```python
from build123d import *

# Parameters (mm, degrees)
SKETCH1_R           = 32.5
BOSS_EXTRUDE1_DEPTH = 2
CUT_EXTRUDE2_DEPTH  = 47.005434462
SKETCH2_R           = 2.5
CUT_EXTRUDE1_DEPTH  = 47.005434462
SKETCH5_R           = 1.5
CUT_EXTRUDE3_DEPTH  = 10


with BuildPart() as part:
    # Sketch1 → Boss-Extrude1 (new body)
    with BuildSketch(Plane(origin=(0, 0, 0), x_dir=(1, 0, 0), z_dir=(0, 1, 0))):
        with Locations(Location((0, 0, 0), (0, 0, 270))):
            Circle(SKETCH1_R)
    extrude(amount=BOSS_EXTRUDE1_DEPTH)

    # Sketch4 → Cut-Extrude2 (cut, through all)
    with BuildSketch(Plane(origin=(0, 2, 0), x_dir=(1, 0, 0), z_dir=(0, 1, 0))):
        with BuildLine():
            Line((-3, -2.645751311), (-3, 2.645751311))
            ThreePointArc((-3, 2.645751311), (4, 0), (-3, -2.645751311))
        make_face()
    extrude(amount=-CUT_EXTRUDE2_DEPTH, mode=Mode.SUBTRACT)

    # Sketch2 → Cut-Extrude1 (cut, through all)
    with BuildSketch(Plane(origin=(0, 2, 0), x_dir=(1, 0, 0), z_dir=(0, 1, 0))):
        with Locations((-30.026084807, -12.437211552)):
            Circle(SKETCH2_R)
        with Locations((-32.5, 0)):
            Circle(SKETCH2_R)
        with Locations((-31.875521613, 6.340435466)):
            Circle(SKETCH2_R)
        with Locations((-30.026084807, 12.437211552)):
            Circle(SKETCH2_R)
        with Locations((-27.0227624, 18.056032573)):
            Circle(SKETCH2_R)
        with Locations((-22.980970389, 22.980970389)):
            Circle(SKETCH2_R)
        with Locations((-18.056032573, 27.0227624)):
            Circle(SKETCH2_R)
        with Locations((-12.437211552, 30.026084807)):
            Circle(SKETCH2_R)
        with Locations((-6.340435466, 31.875521613)):
            Circle(SKETCH2_R)
        with Locations((0, 32.5)):
            Circle(SKETCH2_R)
        with Locations((6.340435466, 31.875521613)):
            Circle(SKETCH2_R)
        with Locations((12.437211552, 30.026084807)):
            Circle(SKETCH2_R)
        with Locations((18.056032573, 27.0227624)):
            Circle(SKETCH2_R)
        with Locations((22.980970389, 22.980970389)):
            Circle(SKETCH2_R)
        with Locations((27.0227624, 18.056032573)):
            Circle(SKETCH2_R)
        with Locations((30.026084807, 12.437211552)):
            Circle(SKETCH2_R)
        with Locations((31.875521613, 6.340435466)):
            Circle(SKETCH2_R)
        with Locations((32.5, 0)):
            Circle(SKETCH2_R)
        with Locations((31.875521613, -6.340435466)):
            Circle(SKETCH2_R)
        with Locations((30.026084807, -12.437211552)):
            Circle(SKETCH2_R)
        with Locations((27.0227624, -18.056032573)):
            Circle(SKETCH2_R)
        with Locations((22.980970389, -22.980970389)):
            Circle(SKETCH2_R)
        with Locations((18.056032573, -27.0227624)):
            Circle(SKETCH2_R)
        with Locations((12.437211552, -30.026084807)):
            Circle(SKETCH2_R)
        with Locations((6.340435466, -31.875521613)):
            Circle(SKETCH2_R)
        with Locations((0, -32.5)):
            Circle(SKETCH2_R)
        with Locations((-6.340435466, -31.875521613)):
            Circle(SKETCH2_R)
        with Locations((-12.437211552, -30.026084807)):
            Circle(SKETCH2_R)
        with Locations((-18.056032573, -27.0227624)):
            Circle(SKETCH2_R)
        with Locations((-22.980970389, -22.980970389)):
            Circle(SKETCH2_R)
        with Locations((-27.0227624, -18.056032573)):
            Circle(SKETCH2_R)
        with Locations((-31.875521613, -6.340435466)):
            Circle(SKETCH2_R)
    extrude(amount=-CUT_EXTRUDE1_DEPTH, mode=Mode.SUBTRACT)

    # Sketch5 → Cut-Extrude3 (cut)
    with BuildSketch(Plane(origin=(0, 2, 0), x_dir=(1, 0, 0), z_dir=(0, 1, 0))):
        with Locations(Location((-25, 0, 0), (0, 0, 270))):
            Circle(SKETCH5_R)
        with Locations(Location((12.5, 21.650635095, 0), (0, 0, 270))):
            Circle(SKETCH5_R)
        with Locations(Location((12.5, -21.650635095, 0), (0, 0, 270))):
            Circle(SKETCH5_R)
    extrude(amount=-CUT_EXTRUDE3_DEPTH, mode=Mode.SUBTRACT)


solid = part.part
```
Here's how the part is built. I have some questions about the finished solid (model axes, mm). Give positions to 0.01 mm unless a question says otherwise; leave off trailing zeros. Order: outer loops, then holes, each group sorted by start corner. A loop starts at its lowest first (then second) coordinate and runs counter-clockwise, first axis right, second up. Notation, with made-up numbers: (-5.5, 22.5) -> (20.5, 22.5) arc R9 ccw to (20.5, 34.5) -> close; hole circle Ø1 at (17, 68.25). An arc over 180 degrees is marked (long way). Use CSV: the item, a comma, the result in double quotes. Start each with the question number.
Item 1: Suppose I cut it at D-D (x = -13.5). List the corners of the cut face in (y, z) for me, and give its area (3 significant figures).
Item 2: Thinking about a two-plate mould opening in Z: for faces 1 (the flat face through (0, 2, 7)), 2 (the cylindrical face through (29.435, 1.014, 5.8)), 3 (the cylindrical face through (0, 1, 30)), which applies, pulls with the +Z half, pulls with the -Z half, needs draft (parallel to the pull), parting line crosses it, or undercut?
Item 3: I'm going to push flat-ended pins straight in: P1, Ø1.8, axis at x = 12.5, z = -21.65, coming from the +Y side; P2, Ø6, axis at x = -12.5, z = -13, coming from the -Y side; P3, Ø0.6, axis at y = 1, z = 0, coming from the +X side. Where does each tip first touch, or does it pass through?
Item 4: Suppose I cut it at C-C (y = 0.55). Give the number of separate pieces and of enclosed holes in the cut face, and give its area (3 significant figures).
Item 5: Suppose I cut it at A-A (z = 0). List the corners of the cut face in (x, y) for me, and give its area (3 significant figures).
Item 6: If I drill on probe 1 along X at (y, z) = (0.9, 0); probe 2 along X at (y, z) = (1.65, 21); probe 3 along Z at (x, y) = (0, 0.85), over which ranges is the centre line in solid material (lowest first)? Write a range as [from, to].
Item 7: Suppose I cut it at B-B (x = 12.5). List the corners of the cut face in (y, z) for me.
Answer block:
1,outline,"(0, -27.76) -> (2, -27.76) -> (2, 27.76) -> (0, 27.76) -> close"
1,area,"111 mm^2"
2,face 1,"needs draft"
2,face 2,"undercut"
2,face 3,"pulls with the +Z half"
3,P1,"passes through"
3,P2,"stops at y = 0"
3,P3,"stops at x = 30.02"
4,separate pieces,"1"
4,enclosed holes,"4"
4,area,"2,940 mm^2"
5,outline,"(-30, 0) -> (-26.5, 0) -> (-26.5, 2) -> (-30, 2) -> close; (-23.5, 0) -> (-3, 0) -> (-3, 2) -> (-23.5, 2) -> close; (4, 0) -> (30, 0) -> (30, 2) -> (4, 2) -> close"
5,area,"100 mm^2"
6,probe 1,"x = [-30, -26.5], [-23.5, -3], [4, 30]"
6,probe 2,"x = [-24.8, -24.51], [-21.46, 11.15], [13.85, 21.46], [24.51, 24.8]"
6,probe 3,"z = [-30, -4], [4, 30]"
7,outline,"(0, -27.53) -> (2, -27.53) -> (2, -23.15) -> (0, -23.15) -> close; (0, -20.15) -> (2, -20.15) -> (2, 20.15) -> (0, 20.15) -> close; (0, 23.15) -> (2, 23.15) -> (2, 27.53) -> (0, 27.53) -> close"
